Solid Edge part; units mm, degrees
sketch "Sketch1" plane through (0, 0, 0) normal (0, -1, 0) x (1, 0, 0)
  line L0 (37, 24) -> (-13, 24)
  line L1 (-13, 24) -> (-13, 74)
  line L2 (-13, 74) -> (-37, 74)
  line L3 (-37, 74) -> (-37, 0)
  line L4 (-37, 0) -> (37, 0)
  line L5 (37, 0) -> (37, 24)
extrude "Protrusion1" add sketch "Sketch1" against normal blind 24
sketch "Sketch2" plane through (-25, 12, 74) normal (0, 0, 1) x (1, 0, 0)
  line L0 (8.5, -8.5) -> (8.5, 8.5)
  line L1 (8.5, 8.5) -> (-8.5, 8.5)
  line L2 (-8.5, 8.5) -> (-8.5, -8.5)
  line L3 (-8.5, -8.5) -> (8.5, -8.5)
extrude "VaciadoExtruido_1" cut sketch "Sketch2" against normal blind 72.5
sketch "Sketch3" plane through (37, 12, 12) normal (1, 0, 0) x (0, 1, 0)
  line L0 (-10.5, 10.5) -> (-10.5, -10.5)
  line L1 (-10.5, -10.5) -> (10.5, -10.5)
  line L2 (10.5, -10.5) -> (10.5, 10.5)
  line L3 (-10.5, 10.5) -> (10.5, 10.5)
extrude "Cutout1" cut sketch "Sketch3" against normal up to surface (70.5 mm away)
sketch "Sketch4" plane through (-13, 12, 49) normal (1, 0, 0) x (0, 0, 1)
  line L0 (25, 4) -> (-25, 4)
  line L1 (-25, 4) -> (-25, -4)
  line L2 (-25, -4) -> (25, -4)
  line L3 (25, 4) -> (25, -4)
extrude "Protrusion2" add sketch "Sketch4" along normal up to surface (50 mm away)
sketch "Sketch5" plane through (12, 8, 49) normal (0, -1, 0) x (0, 0, 1)
  line L0 (5, 25) -> (-25, -5)
  line L1 (-25, -25) -> (-25, -5)
  line L2 (25, -25) -> (-25, -25)
  line L3 (25, 25) -> (25, -25)
  line L4 (5, 25) -> (25, 25)
extrude "Cutout2" cut sketch "Sketch5" against normal through all
chamfer "Chaflán_1" distance 1.25 angle 45 9 edges at (-37, 0, 37) (-37, 24, 37) (-13, 0, 49) (12, 0, 24) (0, 0, 0) (-37, 12, 0) (0, 24, 0) (12, 24, 24) (-13, 24, 49)
sketch "Sketch6" plane through (0.625, 0, 37.625) normal (0, -1, 0) x (1, 0, 0)
  circle A0 centre (-25.625, 21.375) radius 2.25
  circle A1 centre (-25.625, -25.625) radius 2.25
  circle A2 centre (21.375, -25.625) radius 2.25
extrude "Cutout3" cut sketch "Sketch6" against normal through all
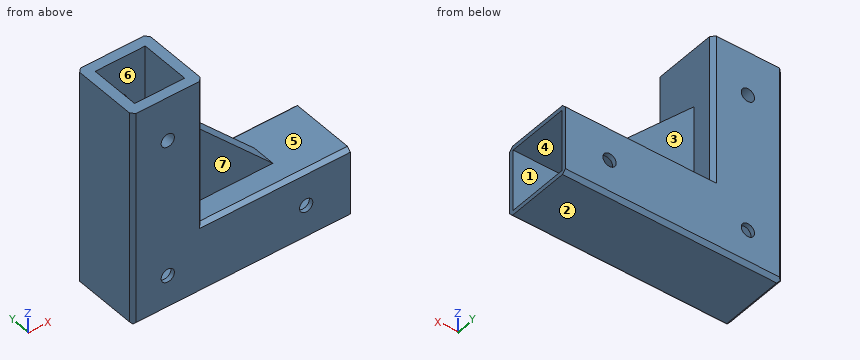
CAD build for the part. Positions are in the model's coordinates, mm. Face numbers are marked on the shaded views. A direction names the side the tool comes from. Coordinates: 2 decimals unless noted, no trailing zeros. Write each loop counter-clockwise with the first axis right and the second up, starting at its lowest first coordinate (ties: lowest second). Pieces come first, ordered by that corner, then holes.
(1) Cut at D-D, the plane z = 12. List the corners of the cut face in (x, y), and give its area (3 significant figures).
(2) Drill centre lines: probe 1 along Z at (x, y) = (-25, 21.95); probe 2 along Z at (x, y) = (-6, 21); probe 3 along Z at (x, y) = (-25, 1.15). Where is each one in solid material? Low to high.
(3) Two-plate mould, pull along Y, no slides. Class the marked faces 1, 2 and 3: +Y half, -Y half, draft (parallel to the pull), parting line (faces both ways), or undercut.
(4) 3-axis set-ups, long thin cutter, end or side, ignore diameter. For the marked faces 4, 5, 6 and 7: which of +Z, -Z, +X, -X, +Y, -Y reach the whole face in a straight line?
(5) Cut at A-A, the plane y = 15. List the corners of the cut face in (x, z).
(6) Cut at B-B, the plane z = 36. List the corners of the cut face in (x, y).
(7) Cut at C-C, the plane x = -25. Count the separate pieces of the cut face and the enclosed holes in it, and give its area (3 significant figures).
(8) Flat gauge pins, fed straight in: pin 1 (8 mm diameter, centred on y = 12, z = 61, fed in from +X); pin 2 (4 mm diameter, centred on x = -25, z = 59, fed in from +Y); pin 3 (11 mm diameter, centred on x = 12, y = 13, fed in from +Z); pin 4 (15 mm diameter, centred on x = -2.5, z = 32, fed in from -Y). Where does each tip first touch, or does it go through?
Geometry says:
1. outline: (-37, 1.25) - (-35.75, 0) - (-27.25, 0) - (-27.25, 1.5) - (-33.5, 1.5) - (-33.5, 22.5) - (-27.25, 22.5) - (-27.25, 24) - (-35.75, 24) - (-37, 22.75) - close; (-22.75, 0) - (19.75, 0) - (19.75, 1.5) - (-22.75, 1.5) - close; (-22.75, 22.5) - (19.75, 22.5) - (19.75, 24) - (-22.75, 24) - close; (24.25, 0) - (37, 0) - (37, 1.5) - (24.25, 1.5) - close; (24.25, 22.5) - (37, 22.5) - (37, 24) - (24.25, 24) - close
1. area: 267 mm2
2. probe 1: z = 0 to 1.5, 22.5 to 56.75, 61.25 to 74
2. probe 2: z = 0 to 1.5, 22.5 to 24
2. probe 3: z = 0.1 to 9.75, 14.25 to 56.75, 61.25 to 74
3. face 1: undercut
3. face 2: draft
3. face 3: +Y half
4. face 4: +X
4. face 5: +Z, +X
4. face 6: +Z
4. face 7: +Z, +X, -Y
5. outline: (-37, 1.25) - (-35.75, 0) - (37, 0) - (37, 1.5) - (-33.5, 1.5) - (-33.5, 74) - (-37, 74) - close; (-16.5, 22.5) - (37, 22.5) - (37, 24) - (17, 24) - (-13, 54) - (-13, 74) - (-16.5, 74) - close
6. outline: (-37, 1.25) - (-35.75, 0) - (-14.25, 0) - (-13, 1.25) - (-13, 8) - (5, 8) - (5, 16) - (-13, 16) - (-13, 22.75) - (-14.25, 24) - (-35.75, 24) - (-37, 22.75) - close; hole (-33.5, 3.5) - (-16.5, 3.5) - (-16.5, 20.5) - (-33.5, 20.5) - close
7. separate pieces: 5
7. enclosed holes: 0
7. area: 413 mm2
8. pin 1: stops at x = -13
8. pin 2: passes through
8. pin 3: stops at z = 34.5
8. pin 4: stops at y = 8
